from build123d import *

# Parameters (mm, degrees)
F1_DEPTH    = 68.58
F2_T1_DEPTH = 116.511978168


# Not quite as in the source:
# - a fillet or chamfer that OpenCascade refuses, or shapes differently, is made with other operations: its cross-section is extruded or revolved along the edge and cut away or added


with BuildPart() as f1:
    # F0 (on Front) → F1 (new body)
    with BuildSketch(Plane.XZ):
        Polygon((-12.7, 0), (0, 0), (0, 28.575), (-50.8, 28.575), (-50.8, 0), (-38.1, 0), (-38.1, 25.4), (-12.7, 25.4), align=None)
    extrude(amount=F1_DEPTH)

    # F2: chamfer of 12.7 x 7.3323484187 on 2 edges, made by hand

    # F2_s2 → F2_t1 (cut)
    with BuildSketch(Plane.YZ.offset(-83.655989084)):
        Polygon((-12.7, 28.575), (0, 21.2426515813), (0, 28.575), align=None)
        Polygon((-55.88, 28.575), (-68.58, 21.2426515813), (-68.58, 28.575), align=None)
    extrude(amount=F2_T1_DEPTH, mode=Mode.SUBTRACT)


solid = f1.part
The listing builds one solid part. Answer for the finished solid, in the listing's coordinates (mm). A direction names the side the tool comes from. Coordinates: 2 decimals unless noted, no trailing zeros. Write each loop counter-clockwise with the first axis right and the second up, starting at its lowest first coordinate (ties: lowest second). Pieces come first, ordered by that corner, then holes. Notation, with made-up numbers: (78.5, 19) - (126.5, 19) arc R27 ccw to (126.5, 46) - close; hole circle Ø3 at (40.25, -5). An arc over 180 degrees is marked (long way). Answer as CSV lines item,"result".
1. Find section A-A (z = 4). Give the vertices of the cut face in (x, y), plus the area to 3 significant figures.
Computed values:
outline,"(-50.8, -68.58) - (-38.1, -68.58) - (-38.1, 0) - (-50.8, 0) - close; (-12.7, -68.58) - (0, -68.58) - (0, 0) - (-12.7, 0) - close"
area,"1,740 mm²"
2. Find section C-C (x = -6). Give the vertices of the cut face in (y, z) (3 decimals), plus the area to 3 significant figures.
Computed values:
outline,"(-68.58, 0) - (0, 0) - (0, 21.243) - (-12.7, 28.575) - (-55.88, 28.575) - (-68.58, 21.243) - close"
area,"1,870 mm²"
3. Straight lines are drawn through the part: line 1 (X direction, y = -15, z = 2.25); line 2 (Z direction, x = -17, y = -53) (3 decimals); line 3 (Z direction, x = -40.5, y = -64.5). For each, find the intervals that lie inside material, in ascending order. Write a range as [from, to].
Computed values:
line 1,"x = [-50.8, -38.1], [-12.7, 0]"
line 2,"z = [25.4, 28.575]"
line 3,"z = [0, 23.6]"
4. A tool of negligible diameter and unlimited length cuts with its end or side. For faces 1 (the flat face through (-26, -34, 25.4)), 2 (the flat face through (-50.8, -34, 14)), from which of +Z, -Z, +X, -X, +Y, -Y can it reach the whole face along a straight path? Write none if from no direction.
Computed values:
face 1,"-Z, +Y, -Y"
face 2,"+Z, -Z, -X, +Y, -Y"
5. Find section D-D (x = -35). Give the vertices of the cut face in (y, z) (3 decimals), plus the area to 3 significant figures.
Computed values:
outline,"(-61.379, 25.4) - (-7.201, 25.4) - (-12.7, 28.575) - (-55.88, 28.575) - close"
area,"155 mm²"
6. Find section B-B (y = -46.5). Give the vertices of the cut face in (x, z) (3 decimals), plus the area to 3 significant figures.
Computed values:
outline,"(-50.8, 0) - (-38.1, 0) - (-38.1, 25.4) - (-12.7, 25.4) - (-12.7, 0) - (0, 0) - (0, 28.575) - (-50.8, 28.575) - close"
area,"806 mm²"
7. Given P1, Ø5, axis at y = -47, z = 18, coming from the +X side; P2, Ø12.5, axis at x = -28.5, y = -43.5, coming from the -Z side, each flat-ended and moving along its own axis, determine where each tip first touches the part or whether it passes through.
Computed values:
P1,"stops at x = 0"
P2,"stops at z = 25.4"
8. Determine the mould class of faces 3 (the flat face through (0, -34, 14)), 4 (the flat face through (-25.756, -60.73, 25.775)), 5 (the flat face through (-38.1, -34, 13)) for opening direction X: +X half, -X half, draft (parallel to the pull), parting line (faces both ways), or undercut.
Computed values:
face 3,"+X half"
face 4,"draft"
face 5,"undercut"
